Geometry: final body of the model. Coordinates: model frame, mm. Face numbers are marked on the shaded views. A direction names the side the tool comes from. Give positions to 0.01 mm unless a question says otherwise; leave off trailing zeros. Write each loop counter-clockwise with the first axis right and the second up, starting at its lowest first coordinate (ties: lowest second). Pieces come first, ordered by that corner, then holes. Notation, with made-up numbers: M 31,87.25 L 43,87.25 A17 cw 43,116.25 Z; hole C 63,85.25 d9. An arc over 180 degrees is marked long. Use a Markdown table: item, result. Add a question column.
(1) Cut plane C-C (x = -12). Output: boundary loops of the cut face in (y, z).
(2) Cut plane B-B (z = 16.5). Output: boundary loops of the cut face in (x, y), plus the area to 3 significant figures.
(3) Material intervals for L1, parallel to X at y = 2.45, z = 14; L2, parallel to Z at x = 6, y = 1.7; L3, parallel to Z at x = 0, y = 2.85, sorted ascending.
(4) Pin query (flat end, axial travel): pin 1 Ø1 at (x, y) = (-6, 1.5) entering from +Z; pin 2 Ø1.6 at (x, y) = (8, 3) entering from +Z; pin 3 Ø2.5 at (y, z) = (3, 16.5) entering from +X. Return the tip coordinate at first contact, or that it passes through.
(5) Reachability of the marked faces 1 and 2 from +Z, -Z, +X, -X, +Y, -Y: full face, straight path, thin tool, end or side. Return the list, or none.
(6) Cut plane A-A (y = 0.45). Output: boundary loops of the cut face in (x, z), plus the area to 3 significant figures.
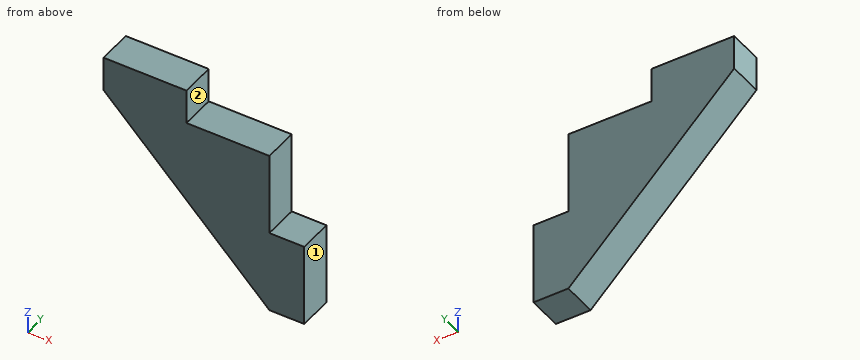
```python
from build123d import *

# Parameters (mm, degrees)
SKETCH1_W           = 12.7
SKETCH1_H           = 5.334
SKETCH1_W_2         = 5.334
SKETCH1_H_2         = 12.7
BOSS_EXTRUDE1_DEPTH = 5.334


with BuildPart() as part:
    # Sketch1 → Boss-Extrude1 (new body)
    with BuildSketch(Plane(origin=(0, 0, 0), x_dir=(1, 0, 0), z_dir=(0, 1, 0))):
        with Locations((-14.711985437, -16.289114223)):
            Rectangle(SKETCH1_W, SKETCH1_H)
        Polygon((4.338014563, 11.777885777), (4.338014563, -13.622114223), (-21.061985437, -13.622114223), align=None)
        with Locations((7.005014563, 5.427885777)):
            Rectangle(SKETCH1_W_2, SKETCH1_H_2)
    extrude(amount=BOSS_EXTRUDE1_DEPTH)


solid = part.part
```
Answer list:
| question | item | result |
|---|---|---|
| 1 | outline | M 0,4.56 L 5.33,4.56 L 5.33,18.96 L 0,18.96 Z |
| 2 | outline | M -21.06,0 L -8.36,0 L -8.36,5.33 L -21.06,5.33 Z |
| 2 | area | 67.7 mm² |
| 3 | L1 | -21.06 to -8.36 |
| 3 | L2 | -11.78 to 0.92 |
| 3 | L3 | -7.44 to 13.62 |
| 4 | pin 1 | z = 13.62 |
| 4 | pin 2 | z = 0.92 |
| 4 | pin 3 | x = -8.36 |
| 5 | face 1 | +Z, -Z, +X, +Y, -Y |
| 5 | face 2 | +Z, +X, +Y, -Y |
| 6 | outline | M -21.06,13.62 L 4.34,-11.78 L 9.67,-11.78 L 9.67,0.92 L 4.34,0.92 L 4.34,13.62 L -8.36,13.62 L -8.36,18.96 L -21.06,18.96 Z |
| 6 | area | 458 mm² |
